For this review, take the finished solid that the model builds, in its own axes (mm). A direction names the side the tool comes from. Round coordinates to 2 decimals unless told otherwise and drop trailing zeros. Order: outer loops, then holes, each group sorted by start corner. A loop starts at its lowest first (then second) coordinate and runs counter-clockwise, first axis right, second up. Notation, with made-up numbers: (-15, 11) - (36, 11) arc R23 ccw to (36, 43) - close; hole circle Ø9 at (15.5, -27). An arc over 180 degrees is marked (long way). One line per question, with ' | ' between items.
```python
from build123d import *

# Parameters (mm, degrees)
SKETCH1_W           = 60
SKETCH1_H           = 40
BOSS_EXTRUDE1_DEPTH = 30
CUT_LOFT2_START     = -14
CUT_LOFT2_DEPTH     = 69
SKETCH9_W           = 30
SKETCH9_H           = 10
CUT_EXTRUDE4_DEPTH  = 50


with BuildPart() as part:
    # Sketch1 → Boss-Extrude1 (new body)
    with BuildSketch(Plane(origin=(0, 0, 0), x_dir=(1, 0, 0), z_dir=(0, 1, 0))):
        with Locations((30, 20)):
            Rectangle(SKETCH1_W, SKETCH1_H)
    extrude(amount=BOSS_EXTRUDE1_DEPTH)

    # Cut-Loft2: read off the stored shape, not the designer's step
    # Cut-Loft2 outline → Cut-Loft2 (cut)
    with BuildSketch(Plane(origin=(0, 0, 0), x_dir=(0.4472135954999584, 0.8944271909999156, 0), z_dir=(0.8944271909999156, -0.4472135954999584, 0)).offset(CUT_LOFT2_START)):
        Polygon((55, 0), (26.83281573, 0), (53.66563146, -40), (54.336451853, -41), (55, -41), align=None)
    extrude(amount=CUT_LOFT2_DEPTH, mode=Mode.SUBTRACT)

    # Sketch9 → Cut-Extrude4 (cut)
    with BuildSketch(Plane(origin=(0, 30, 0), x_dir=(1, 0, 0), z_dir=(0, 1, 0))):
        with Locations((30, 20)):
            Rectangle(SKETCH9_W, SKETCH9_H)
    extrude(amount=-CUT_EXTRUDE4_DEPTH, mode=Mode.SUBTRACT)


solid = part.part
```
(1) Insertion check: pin 1 (6 mm diameter, centred on x = 35.5, z = -5.5, fed in from +Y); pin 2 (6 mm diameter, centred on x = 37.5, y = 22.5, fed in from +Z). Each pin has a flat end and moves straight along its axis. Give the tip position at first contact, or say it passes through.
Output values:
pin 1: y = 19.08 | pin 2: z = -10.53
(2) For faces 1 (the flat face through (0, 15, -20)), 2 (the flat face through (45, 10, -20)), list the 3-axis set-ups (+Z, -Z, +X, -X, +Y, -Y) from which the entire face can be reached by the end or side of a thin tool; tool diameter is ignored.
Output values:
face 1: +Z, -Z, -X, +Y, -Y | face 2: +Y, -Y
(3) We need section A-A on x = 32. State the section outline as (y, z) points, plus the area to 3 significant figures.
Output values:
outline: (0, -40) - (30, -40) - (30, -25) - (0, -25) - close; (0, -15) - (25.25, -15) - (14, 0) - (0, 0) - close | area: 744 mm^2
(4) We need section C-C on y = 15. State the section outline as (x, z) points.
Output values:
outline: (0, -40) - (60, -40) - (60, -20) - (30, 0) - (0, 0) - close; hole (15, -25) - (45, -25) - (45, -15) - (15, -15) - close
(5) Mouldability with a two-part tool opening along X and no side actions: class faces 3 (the flat face through (30, 12, -15)), 4 (the flat face through (23, 30, -29)), 5 (the flat face through (60, 8, -29)) as released by +X, released by -X, zero draft, split by the parting line, or undercut.
Output values:
face 3: undercut | face 4: zero draft | face 5: released by +X
(6) We need section B-B on z = -21. State the section outline as (x, y) points, plus the area to 4 significant figures.
Output values:
outline: (0, 0) - (15, 0) - (15, 30) - (0, 30) - close; (45, 0) - (60, 0) - (60, 15.75) - (45, 23.25) - close | area: 742.5 mm^2
(7) We need section D-D on y = 22.5. State the section outline as (x, z) points, plus the area to 3 significant figures.
Output values:
outline: (0, -40) - (60, -40) - (60, -30) - (45, -20) - (45, -25) - (15, -25) - (15, -15) - (37.5, -15) - (15, 0) - (0, 0) - close | area: 1,440 mm^2
(8) For probe 1 along Z at (x, y) = (36.5, 10.5); probe 2 along X at (y, z) = (3.5, -19.5); probe 3 along X at (y, z) = (29.5, -17), list the stretches that pass through material, from the lowest coordinate up. Write a range as [from, to].
Output values:
probe 1: [-40, -25], [-15, 0] | probe 2: [0, 15], [45, 60] | probe 3: [0, 15]
